```python
from build123d import *

# Parameters (mm, degrees)
SKETCH1_R           = 5.4102
BOSS_EXTRUDE1_DEPTH = 5.715
SKETCH2_R           = 3.9243
BOSS_EXTRUDE2_DEPTH = 25.4
SKETCH3_W           = 9.007282867
SKETCH3_H           = 9.525
CUT_EXTRUDE1_DEPTH  = 2.54


with BuildPart() as part:
    # Sketch1 → Boss-Extrude1 (new body)
    with BuildSketch(Plane.XY):
        Circle(SKETCH1_R)
    extrude(amount=BOSS_EXTRUDE1_DEPTH)

    # Sketch2 → Boss-Extrude2 (add)
    with BuildSketch(Plane(origin=(0, 0, 0), x_dir=(-1, 0, 0), z_dir=(0, 0, -1))):
        with Locations(Location((0, 0, 0), (0, 0, 180))):
            Circle(SKETCH2_R)
    extrude(amount=BOSS_EXTRUDE2_DEPTH)

    # Sketch3 → Cut-Extrude1 (cut)
    with BuildSketch(Plane(origin=(0, 3.9243, 0), x_dir=(1, 0, 0), z_dir=(0, 1, 0))):
        with Locations((-0.278552297, 17.4625)):
            Rectangle(SKETCH3_W, SKETCH3_H)
    extrude(amount=-CUT_EXTRUDE1_DEPTH, mode=Mode.SUBTRACT)


solid = part.part
```
The model under review builds one solid part; all positions refer to its coordinate system, in mm. A direction names the side the tool comes from. Round coordinates to 2 decimals unless told otherwise and drop trailing zeros. Loops run counter-clockwise (first coordinate to the right, second up) from the corner with the lowest first, then second, coordinate; pieces in that order, holes last. Notation, with made-up numbers: M 6,37 L 13,37 A34 cw 13,71 Z; hole C 19.5,82.5 d7. An arc over 180 degrees is marked long. Answer as a JSON object with one key per item and string values.
(1) Tool access review of faces 5 (the flat face through (4, 2, 0)), 6 (the flat face through (0, 2, -22.225)), 7 (the cylindrical face through (5.16, 1.63, 2.82)): name each direction out of +Z, -Z, +X, -X, +Y, -Y from which nothing blocks a thin tool from reaching the whole face with its end or side.
Resolved:
{"face 5": "-Z", "face 6": "+X, -X, +Y", "face 7": "+Z, -Z"}
(2) Clearance check with flat-ended pins moving along their axes: P1, Ø2, axis at x = -1, z = -18.5, coming from the +Y side; P2, Ø4, axis at y = 2.5, z = 1, coming from the +X side; P3, Ø2, axis at x = -2, z = -0.5, coming from the -Y side. State where each tip first meets the part, or that it passes through.
Resolved:
{"P1": "y = 1.38", "P2": "x = 5.39", "P3": "y = -5.29"}
(3) Draft analysis for pull direction Z (two halves, no side actions). For faces 1 (the flat face through (0, 0, 5.715)), 2 (the flat face through (0, 2, -12.7)), 3 (the cylindrical face through (-0.51, -3.89, -12.52)), 4 (the flat face through (0, 0, -25.4)), state which applies: released by +Z, released by -Z, zero draft, split by the parting line, or undercut.
Resolved:
{"face 1": "released by +Z", "face 2": "undercut", "face 3": "zero draft", "face 4": "released by -Z"}
(4) To check wall thickness, follow line 1 along Z through (x, y) = (-1, 3) (3 decimals); line 2 along Z through (x, y) = (4, 1) (3 decimals); line 3 along X through (y, z) = (-3.25, -5.5). State the ranges of each line that lie inside material, in increasing order.
Resolved:
{"line 1": "-25.4 to -22.225, -12.7 to 5.715", "line 2": "0 to 5.715", "line 3": "-2.2 to 2.2"}
(5) Take a section at A-A on y = 3. Give the boundary of the cut face in (x, z) (3 decimals), and give its area (3 significant figures).
Resolved:
{"outline": "M -4.502,0 L -2.53,0 L -2.53,-12.7 L 2.53,-12.7 L 2.53,0 L 4.502,0 L 4.502,5.715 L -4.502,5.715 Z; M -2.53,-25.4 L 2.53,-25.4 L 2.53,-22.225 L -2.53,-22.225 Z", "area": "132 mm²"}
(6) Take a section at B-B on y = 0. Give the boundary of the cut face in (x, z) (3 decimals), and give its area (3 significant figures).
Resolved:
{"outline": "M -5.41,0 L -3.924,0 L -3.924,-25.4 L 3.924,-25.4 L 3.924,0 L 5.41,0 L 5.41,5.715 L -5.41,5.715 Z", "area": "261 mm²"}
(7) Take a section at C-C on x = 0. Give the boundary of the cut face in (y, z) (3 decimals), and give its area (3 significant figures).
Resolved:
{"outline": "M -5.41,0 L -3.924,0 L -3.924,-25.4 L 3.924,-25.4 L 3.924,-22.225 L 1.384,-22.225 L 1.384,-12.7 L 3.924,-12.7 L 3.924,0 L 5.41,0 L 5.41,5.715 L -5.41,5.715 Z", "area": "237 mm²"}
(8) Take a section at D-D on z = -16. Give the boundary of the cut face in (x, y).
Resolved:
{"outline": "M -3.67,1.38 A3.92 ccw long 3.67,1.38 Z"}
